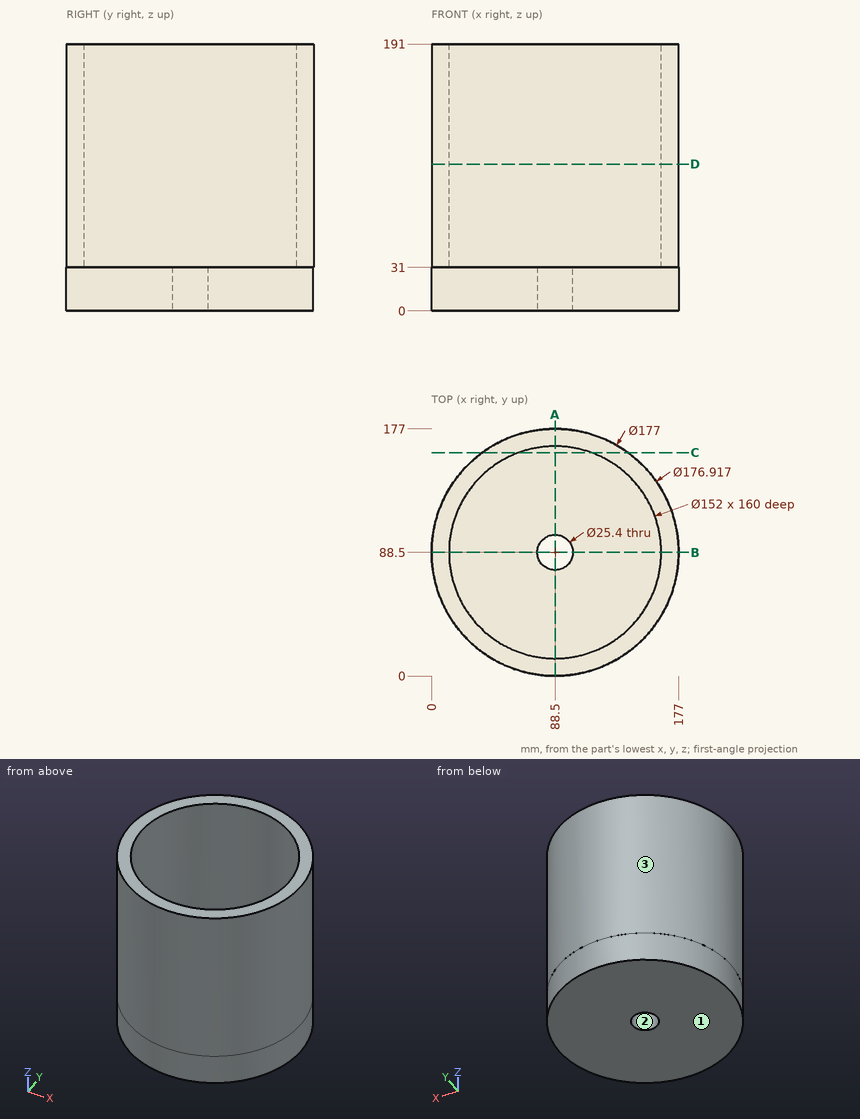
Source: three-view drawing plus pictorial views. Frame: mm from the lowest corner of the part. Give positions to 0.01 mm unless a question says otherwise; leave off trailing zeros. Write each loop counter-clockwise with the first axis right and the second up, starting at its lowest first coordinate (ties: lowest second). Pieces come first, ordered by that corner, then holes. Notation, with made-up numbers: (20.25, 84) - (59.25, 84) arc R21 cw to (59.25, 94) - close; hole circle Ø7 at (-12, 7.25). An arc over 180 degrees is marked (long way). Write item = value, one per line. Start each with the question number.
Q1. Pin query (flat end, axial travel): pin 1 Ø2 at (x, y) = (93, 111) entering from +Z; pin 2 Ø3 at (x, z) = (121.5, 68) entering from +Y (1 decimal); pin 3 Ø5 at (y, z) = (19, 33.5) entering from -X. Return the tip coordinate at first contact, or that it passes through.
Q2. Material intervals for probe 1 along Y at (x, z) = (88, 16); probe 2 along Y at (x, z) = (88, 70); probe 3 along X at (y, z) = (88.5, 17), sorted ascending.
Q3. Draft query along X for the marked faces 1, 2 and 3. Return one class per face: +X half, -X half, draft (parallel to the pull), parting line (faces both ways), or undercut.
Q4. Cut plane A-A, the plane x = 88.5. Return loops of the section in (y, z), then the cut area to 3 significant figures.
Q5. Cut plane C-C, the plane y = 160. Return loops of the section in (x, z), then the cut area to 3 significant figures.
Q6. Cut plane D-D, the plane z = 105. Return loops of the section in (x, y).
Computed values:
q1.pin_1 = 31
q1.pin_2 = 171.2
q1.pin_3 = 30.68
q2.probe_1 = 0.04 to 75.81, 101.19 to 176.96
q2.probe_2 = 0 to 12.5, 164.5 to 177
q2.probe_3 = 0.04 to 75.8, 101.2 to 176.96
q3.face_1 = draft
q3.face_2 = undercut
q3.face_3 = parting line
q4.outline = (0, 31) - (0.04, 31) - (0.04, 0) - (75.8, 0) - (75.8, 31) - (12.5, 31) - (12.5, 191) - (0, 191) - close; (101.2, 0) - (176.96, 0) - (176.96, 31) - (177, 31) - (177, 191) - (164.5, 191) - (164.5, 31) - (101.2, 31) - close
q4.area = 8,700 mm²
q5.outline = (36.35, 31) - (36.42, 31) - (36.42, 0) - (140.58, 0) - (140.58, 31) - (140.65, 31) - (140.65, 191) - (114.26, 191) - (114.26, 31) - (62.74, 31) - (62.74, 191) - (36.35, 191) - close
q5.area = 11,700 mm²
q6.outline = circle Ø177 at (88.5, 88.5); hole circle Ø152 at (88.5, 88.5)
